```python
from build123d import *

# Parameters (mm, degrees)
F2_DEPTH = 107.95
F3_DEPTH = 19.05
F4_DEPTH = 19.05
F1_R     = 44.45
F5_DEPTH = 127
F6_DEPTH = 152.4


# Not quite as in the source:
# - a variable given as a bare number and used for a length is read in inches; the dataset says mm whatever the document's units were


with BuildPart() as f2:
    # F1 (on Front) → F2 (new body)
    with BuildSketch(Plane.XZ):
        with BuildLine():
            Line((118.745, 140.2388613905), (118.745, 50.8))
            Line((118.745, 50.8), (135.255, 50.8))
            Line((135.255, 50.8), (135.255, 140.2388613905))
            ThreePointArc((135.255, 140.2388613905), (127, 139.7), (118.745, 140.2388613905))
        make_face()
    extrude(amount=F2_DEPTH)

    # F1 (on Front) → F3 (join)
    with BuildSketch(Plane.XZ):
        with BuildLine():
            Line((135.255, 50.8), (254, 50.8))
            Line((254, 50.8), (186.2277468166, 226.0981223472))
            ThreePointArc((186.2277468166, 226.0981223472), (189.4228000127, 214.8466320699), (190.5, 203.2))
            ThreePointArc((190.5, 203.2), (174.7307160013, 161.3188735825), (135.255, 140.2388613905))
            Line((135.255, 140.2388613905), (135.255, 50.8))
        make_face()
    extrude(amount=F3_DEPTH)

    # F1 (on Front) → F4 (join)
    with BuildSketch(Plane.XZ):
        with BuildLine():
            Line((67.7722531834, 226.0981223472), (0, 50.8))
            Line((0, 50.8), (118.745, 50.8))
            Line((118.745, 50.8), (118.745, 140.2388613905))
            ThreePointArc((118.745, 140.2388613905), (72.3974959138, 170.7836993549), (67.7722531834, 226.0981223472))
        make_face()
    extrude(amount=F4_DEPTH)

    # F1 (on Front) → F5 (join)
    with BuildSketch(Plane.XZ):
        with BuildLine():
            ThreePointArc((186.2277468166, 226.0981223472), (127, 266.7), (67.7722531834, 226.0981223472))
            ThreePointArc((67.7722531834, 226.0981223472), (72.3974959138, 170.7836993549), (118.745, 140.2388613905))
            ThreePointArc((118.745, 140.2388613905), (127, 139.7), (135.255, 140.2388613905))
            ThreePointArc((135.255, 140.2388613905), (174.7307160013, 161.3188735825), (190.5, 203.2))
            ThreePointArc((190.5, 203.2), (189.4228000127, 214.8466320699), (186.2277468166, 226.0981223472))
        make_face()
        with Locations((127, 203.2)):
            Circle(F1_R, mode=Mode.SUBTRACT)
    extrude(amount=F5_DEPTH)

    # F1 (on Front) → F6 (join)
    with BuildSketch(Plane.XZ):
        Polygon((0, 50.8), (0, 0), (254, 0), (254, 50.8), (135.255, 50.8), (118.745, 50.8), align=None)
    extrude(amount=F6_DEPTH)


solid = f2.part
```
Model file for the job. Use its own axes, mm. A direction names the side the tool comes from. Coordinates: 2 decimals unless noted, no trailing zeros. Write each loop counter-clockwise with the first axis right and the second up, starting at its lowest first coordinate (ties: lowest second). Pieces come first, ordered by that corner, then holes. Notation, with made-up numbers: (-9, -33) - (47, -33) arc R19 cw to (47, -18) - close; hole circle Ø10 at (31, 83.5). An arc over 180 degrees is marked (long way). One line per item, written item: value. Start each with the question number.
1. Slice it at C-C (z = 180). Write the cut outline in (x, y), plus the area to 3 significant figures.
2. Mould opens along Z. For faces 1 (the flat face through (220.59, -9.39, 137.22)), 2 (the flat face through (72, -19.05, 101)), 3 (the flat face through (84, -127, 190)) say: released by +Z, released by -Z, zero draft, split by the parting line, or undercut.
3. Slice it at B-B (x = 127). Write the cut outline in (y, z).
4. Flat gauge pins, fed straight in: pin 1 (5 mm diameter, centred on x = 128, z = 81.5, fed in from -Y); pin 2 (4 mm diameter, centred on x = 187, y = -26, fed in from +Z); pin 3 (5 mm diameter, centred on y = -62.5, z = 202.5, fed in from -X). Where does each tip first touch, or does it go through?
5. Slice it at A-A (y = -60). Write the cut outline in (x, z) (3 decimals).
6. Slice it at D-D (z = 133.5). Write the cut outline in (x, y) (3 decimals).
7. Tool access for faces 4 (the flat face through (129, -114, 50.8)), 5 (the flat face through (127, -107.95, 96)), 6 (the flat face through (118.745, -63, 96)), 7 (the flat face through (181, -19.05, 101)): list every direction of +Z, -Z, +X, -X, +Y, -Y with a clear straight run to the whole face (end or side of a thin tool).
8. Probe line 1 (Z direction, x = 127, y = -71.5); line 2 (X direction, y = -40, z = 203.5); line 3 (Z direction, x = 162.5, y = -81). List the from-to ranges inside material, lowest first. Write a range as from..to.
Answers below:
1. outline: (49.95, -19.05) - (67.89, -19.05) - (67.89, -127) - (89.08, -127) - (89.08, 0) - (49.95, 0) - close; (164.92, -127) - (186.11, -127) - (186.11, -19.05) - (204.05, -19.05) - (204.05, 0) - (164.92, 0) - close
1. area: 6,070 mm^2
2. face 1: released by +Z
2. face 2: undercut
2. face 3: zero draft
3. outline: (-152.4, 0) - (0, 0) - (0, 158.75) - (-127, 158.75) - (-127, 139.7) - (-107.95, 139.7) - (-107.95, 50.8) - (-152.4, 50.8) - close; (-127, 247.65) - (0, 247.65) - (0, 266.7) - (-127, 266.7) - close
4. pin 1: stops at y = -107.95
4. pin 2: stops at z = 229.05
4. pin 3: stops at x = 63.5
5. outline: (0, 0) - (254, 0) - (254, 50.8) - (135.255, 50.8) - (135.255, 140.239) arc R63.5 ccw (long way) to (118.745, 140.239) - (118.745, 50.8) - (0, 50.8) - close; hole circle Ø88.9 at (127, 203.2)
6. outline: (31.973, -19.05) - (118.745, -19.05) - (118.745, -107.95) - (135.255, -107.95) - (135.255, -19.05) - (222.027, -19.05) - (222.027, 0) - (31.973, 0) - close
7. face 4: -Y
7. face 5: +X, -X, -Y
7. face 6: -X, -Y
7. face 7: +X, -Y
8. line 1: z = 0..158.75, 247.65..266.7
8. line 2: x = 63.5..82.55, 171.45..190.5
8. line 3: z = 0..50.8, 150.55..176.45, 229.95..255.85
